The listing builds one solid part. Answer for the finished solid, in the listing's coordinates (mm). A direction names the side the tool comes from. Give positions to 0.01 mm unless a question says otherwise; leave off trailing zeros. Order: outer loops, then holes, each group sorted by start corner. A loop starts at its lowest first (then second) coordinate and runs counter-clockwise, first axis right, second up.
```python
from build123d import *

# Parameters (mm, degrees)
SKETCH2_W               = 110
SKETCH2_H               = 80
SKETCH2_W_2             = 96
SKETCH2_H_2             = 66
BOSS_EXTRUDE2_DEPTH     = 6
FILLET1_R               = 2.5
SKETCH3_R               = 1.5
CUT_EXTRUDE1_DEPTH      = 136.876166867
FILLET2_R               = 2.5
CUT_EXTRUDE2_DEPTH      = 136.876166867
CUT_EXTRUDE2_DEPTH_BACK = 136.876166867
FILLET3_R               = 5


with BuildPart() as part:
    # Sketch2 → Boss-Extrude2 (new body)
    with BuildSketch(Plane.XY):
        with Locations((-54.66463752, 40)):
            Rectangle(SKETCH2_W, SKETCH2_H)
        with Locations((-54.66463752, 40)):
            Rectangle(SKETCH2_W_2, SKETCH2_H_2, mode=Mode.SUBTRACT)
    extrude(amount=BOSS_EXTRUDE2_DEPTH)

    # Fillet1
    fillet1_edges = [part.edges().sort_by_distance(p)[0] for p in [
        (-6.66463752, 7, 3),
        (-6.66463752, 73, 3),
        (-102.66463752, 73, 3),
        (-102.66463752, 7, 3),
    ]]
    fillet(fillet1_edges, radius=FILLET1_R)

    # Sketch3 → Cut-Extrude1 (cut, through all)
    with BuildSketch(Plane.XY.offset(6)):
        with Locations((-4.66463752, 75)):
            Circle(SKETCH3_R)
        with Locations((-4.66463752, 5)):
            Circle(SKETCH3_R)
        with Locations((-104.66463752, 5)):
            Circle(SKETCH3_R)
        with Locations((-104.66463752, 75)):
            Circle(SKETCH3_R)
    extrude(amount=-CUT_EXTRUDE1_DEPTH, mode=Mode.SUBTRACT)

    # Fillet2
    fillet2_edges = [part.edges().sort_by_distance(p)[0] for p in [
        (0.33536248, 0, 3),
        (-109.66463752, 0, 3),
        (-109.66463752, 80, 3),
        (0.33536248, 80, 3),
    ]]
    fillet(fillet2_edges, radius=FILLET2_R)

    # Sketch4 → Cut-Extrude2 (cut, two sides: drawn at the far end of the back side and taken through both)
    with BuildSketch(Plane(origin=(0, 0, 0), x_dir=(-1, 0, 0), z_dir=(0, 0, -1)).offset(-CUT_EXTRUDE2_DEPTH_BACK)):
        Polygon((29.236938862, -234.527844878), (30.900112939, 0), (30.949754032, 7), (50.799101604, 7), (50.799101604, 0), (50.799101604, -234.533742073), (50.670812865, -703.601208677), (29.108650122, -703.595311481), align=None)
    extrude(amount=CUT_EXTRUDE2_DEPTH + CUT_EXTRUDE2_DEPTH_BACK, mode=Mode.SUBTRACT)

    # Fillet3
    fillet3_edges = [part.edges().sort_by_distance(p)[0] for p in [
        (-30.900112939, 0, 3),
        (-50.799101604, 0, 3),
    ]]
    fillet(fillet3_edges, radius=FILLET3_R)


solid = part.part
```
1) Find section A-A (y = 75). Write down the section's boundary in (x, z), then the cut area to 3 significant figures.
Geometry says:
outline: (-109.66, 0) - (-106.16, 0) - (-106.16, 6) - (-109.66, 6) - close; (-103.16, 0) - (-6.16, 0) - (-6.16, 6) - (-103.16, 6) - close; (-3.16, 0) - (0.34, 0) - (0.34, 6) - (-3.16, 6) - close
area: 624 mm2
2) Straight lines are drawn through the part: probe 1 along X at (y, z) = (75, 2.9); probe 2 along X at (y, z) = (16, 1.4); probe 3 along Y at (x, z) = (-26, 2.4). For each, find the intervals that lie inside material, in ascending order.
Geometry says:
probe 1: x = -109.66 to -106.16, -103.16 to -6.16, -3.16 to 0.34
probe 2: x = -109.66 to -102.66, -6.66 to 0.34
probe 3: y = 0 to 7, 73 to 80
3) A tool of negligible diameter and unlimited length cuts with its end or side. For faces 1 (the flat face through (-55, 80, 3)), 2 (the flat face through (-20, 7, 3)), 3 (the cylindrical face through (-52.225, 1.504, 2.958)), from which of +Z, -Z, +X, -X, +Y, -Y can it reach the whole face along a straight path? Write none if from no direction.
Geometry says:
face 1: +Z, -Z, +X, -X, +Y
face 2: +Z, -Z
face 3: +Z, -Z, -Y
4) Given P1, Ø1.8, axis at x = -104.66, y = 5, coming from the +Z side, flat-ended and moving along its own axis, determine where the tip first touches the part or whether it passes through.
Geometry says:
P1: passes through
5) Find section B-B (z = 2.4). Write down the section's boundary in (x, y), then the cut area to 3 significant figures.
Geometry says:
outline: (-109.66, 2.5) arc R2.5 ccw to (-107.16, 0) - (-55.8, 0) arc R5 ccw to (-50.8, 5) - (-50.8, 7) - (-100.16, 7) arc R2.5 cw to (-102.66, 9.5) - (-102.66, 70.5) arc R2.5 cw to (-100.16, 73) - (-9.16, 73) arc R2.5 cw to (-6.66, 70.5) - (-6.66, 9.5) arc R2.5 cw to (-9.16, 7) - (-30.95, 7) - (-30.94, 4.96) arc R5 ccw to (-25.94, 0) - (-2.16, 0) arc R2.5 ccw to (0.34, 2.5) - (0.34, 77.5) arc R2.5 ccw to (-2.16, 80) - (-107.16, 80) arc R2.5 ccw to (-109.66, 77.5) - close; hole circle Ø3 at (-104.66, 5); hole circle Ø3 at (-104.66, 75); hole circle Ø3 at (-4.66, 5); hole circle Ø3 at (-4.66, 75)
area: 2,290 mm2
6) For a pull along X with two mould halves and no side action, classify faces 4 (the flat face through (-14, 0, 3)), 5 (the cylindrical face through (-101.9, 72.3, 3)), 6 (the flat face through (-109.665, 39, 3)) as +X half, -X half, draft (parallel to the pull), parting line (faces both ways), or undercut.
Geometry says:
face 4: draft
face 5: undercut
face 6: -X half
